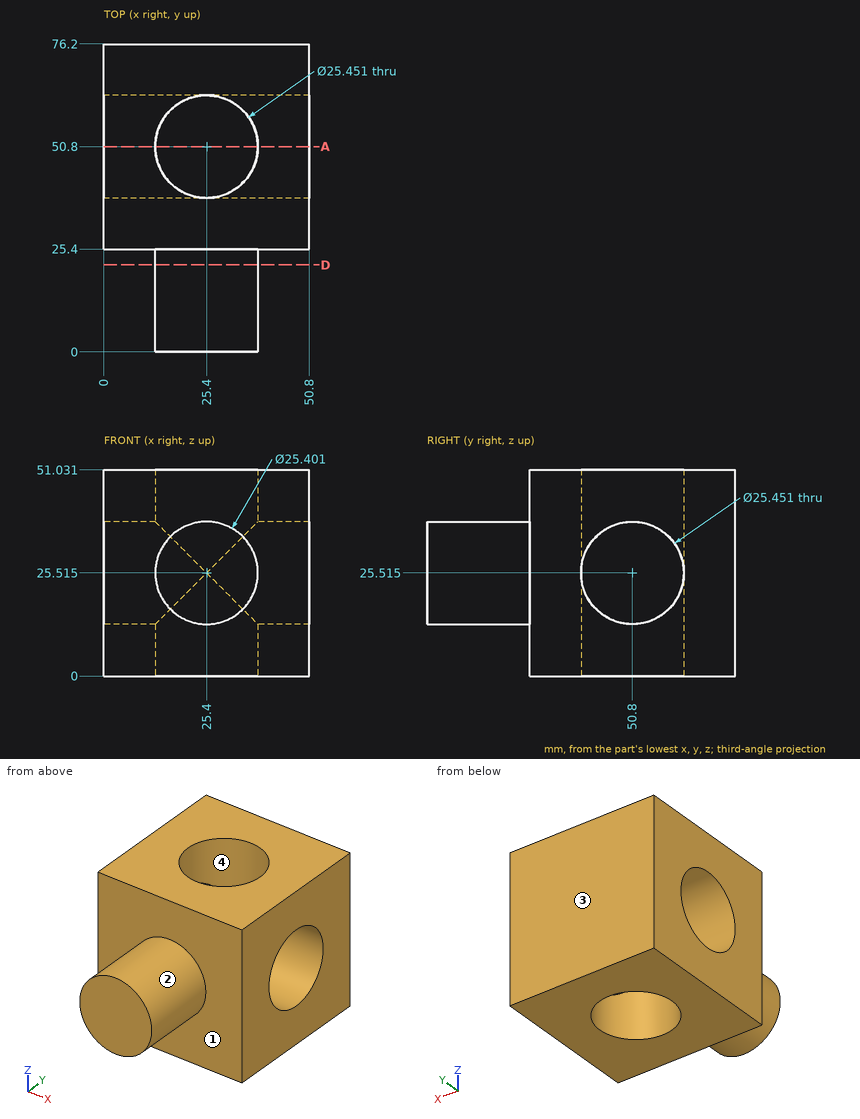
Design review of the part shown in the three views and the two pictorial views. Dimensions are in mm from the part's minimum x, y and z. Round coordinates to 2 decimals unless told otherwise and drop trailing zeros. Loops run counter-clockwise (first coordinate to the right, second up) from the corner with the lowest first, then second, coordinate; pieces in that order, holes last. Notation, with made-up numbers: (28, -18.5) -> (41, -18.5) arc R25 ccw to (41, 11.5) -> close; hole circle Ø4 at (-22, 15). An arc over 180 degrees is marked (long way). Return JSON: item names as keys, results as strings.
(1) For pin 1 (1 mm diameter, centred on y = 8.5, z = 29.5, fed in from -X); pin 2 (10 mm diameter, centred on y = 18, z = 16, fed in from -X); pin 3 (3 mm diameter, centred on x = 25, y = 22, fed in from +Z), all flat-tipped, find the tip position at first contact; note any pin that passes through.
Solved:
{"pin 1": "x = 13.19", "pin 2": "x = 13.53", "pin 3": "z = 38.22"}
(2) Add section D-D on y = 21.5. Write out the cut boundary in (x, z) (1 decimal).
Solved:
{"outline": "circle Ø25.4 at (25.4, 25.5)"}
(3) Add section A-A on y = 50.8. Write out the cut boundary in (x, z) (1 decimal).
Solved:
{"outline": "(0, 0) -> (12.7, 0) -> (12.7, 12.8) -> (0, 12.8) -> close; (0, 38.2) -> (12.7, 38.2) -> (12.7, 51) -> (0, 51) -> close; (38.1, 0) -> (50.8, 0) -> (50.8, 12.8) -> (38.1, 12.8) -> close; (38.1, 38.2) -> (50.8, 38.2) -> (50.8, 51) -> (38.1, 51) -> close"}
(4) For line 1 (Y direction, x = 26, z = 21.5); line 2 (X direction, y = 50, z = 42); line 3 (X direction, y = 40, z = 41.5), list the stretches that pass through material, from the lowest coordinate up.
Solved:
{"line 1": "0 to 38.09, 63.51 to 76.2", "line 2": "0 to 12.7, 38.1 to 50.8", "line 3": "0 to 18.67, 32.13 to 50.8"}
(5) The part is to be moulded in two halves that separate along Y. For the marked faces 1, 2, 3 and 4, say which applies: released by +Y, released by -Y, zero draft, split by the parting line, or undercut.
Solved:
{"face 1": "released by -Y", "face 2": "zero draft", "face 3": "released by +Y", "face 4": "undercut"}
